Part model, mm, in its own coordinate system. Face numbers are marked on the shaded views. A direction names the side the tool comes from. Give positions to 0.01 mm unless a question says otherwise; leave off trailing zeros. Order: outer loops, then holes, each group sorted by start corner. A loop starts at its lowest first (then second) coordinate and runs counter-clockwise, first axis right, second up. Notation, with made-up numbers: M -9.5,59.25 L 16.5,59.25 A19 ccw 16.5,91.25 Z; hole C 47.5,-17.75 d5. An arc over 180 degrees is marked long. Return JSON: item names as keys, results as strings.
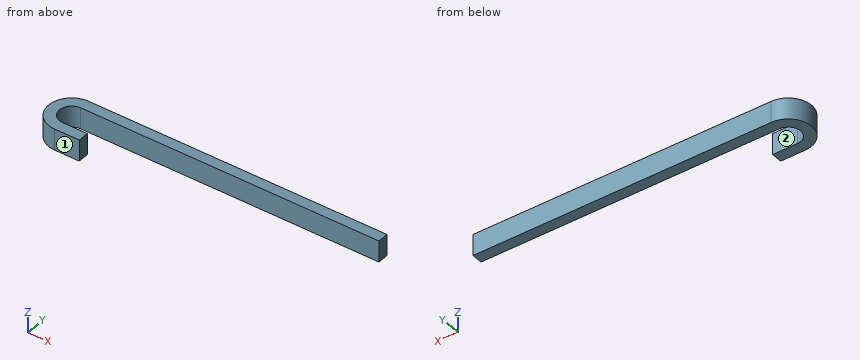
Autodesk Inventor part; units mm, degrees
ref_plane "YZ Plane" through (0, 0, 0) normal (1, 0, 0) x (0, 1, 0)
ref_plane "XZ Plane" through (0, 0, 0) normal (0, 1, 0) x (-1, 0, 0)
ref_plane "XY Plane" through (0, 0, 0) normal (0, 0, 1) x (1, 0, 0)
sketch "Sketch1" plane through (0, 0, 0) normal (0, 0, 1) x (1, 0, 0)
  circle A0 centre (0, 0) radius 42.5
  line L0 (0, -42.5) -> (45.5, -42.5)
  line L1 (45.5, -42.5) -> (45.5, -22.5)
  line L2 (45.5, -22.5) -> (0, -22.5)
  line L3 (0, -22.5) -> (0, -42.5)
  line L4 (0, 42.5) -> (550, 42.5)
  line L5 (550, 42.5) -> (550, 22.5)
  line L6 (550, 22.5) -> (0, 22.5)
  line L7 (0, 22.5) -> (0, 42.5)
  circle A1 centre (0, 0) radius 22.5
  point P0 (0, -22.5)
  point P1 (0, 22.5)
  point P2 (15.5, -22.5)
  point P3 (-42.5, 0)
  dimension "d0" = 85
  dimension "d1" = 20
  dimension "d2" = 20
  dimension "d9" = 550
  dimension "d10" = 58
  dimension "d11" = 30
extrude "Extrusion1" add sketch "Sketch1" along normal blind 39 contours L7 A1 L3 A0 | L4 L5 L6 A0 | A0 L6 L7 | L3 L2 A0 | A0 L2 L1 L0
properties part number "J15BF.1.30_Zaxis"
Q1. Band-saw the part on B-B (z = 33). Give the cut face in (x, y).
Established:
{"outline": "M 0,-42.5 L 45.5,-42.5 L 45.5,-22.5 L 0,-22.5 A22.5 cw 0,22.5 L 550,22.5 L 550,42.5 L 0,42.5 A42.5 ccw Z"}
Q2. Pin check, flat tips, straight feed: pin 1 (19.5 mm diameter, centred on x = 265.5, z = 16, fed in from -Y); pin 2 (1.5 mm diameter, centred on y = -15.5, z = 7.5, fed in from -X); pin 3 (6 mm diameter, centred on y = -36, z = 15, fed in from +X). Stop position of each tip, or through.
Established:
{"pin 1": "stops at y = 22.5", "pin 2": "stops at x = -39.86", "pin 3": "stops at x = 45.5"}
Q3. Band-saw the part on D-D (x = 162). Give the cut face in (y, z).
Established:
{"outline": "M 22.5,0 L 42.5,0 L 42.5,39 L 22.5,39 Z"}
Q4. Band-saw the part on C-C (y = 0). Give the cut face in (x, z), then the cut area to 3 significant figures.
Established:
{"outline": "M -42.5,0 L -22.5,0 L -22.5,39 L -42.5,39 Z", "area": "780 mm²"}
Q5. Probe line 1 along Y through (x, z) = (13.5, 31.5); line 2 along Y through (x, z) = (343.5, 3); line 3 along X through (y, z) = (19, 22). List the from-to ranges inside material, lowest first.
Established:
{"line 1": "y = -42.5 to -22.5, 22.5 to 42.5", "line 2": "y = 22.5 to 42.5", "line 3": "x = -38.02 to -12.05"}
Q6. Band-saw the part on A-A (x = 35.5). Give the cut face in (y, z), then the cut area to 3 significant figures.
Established:
{"outline": "M -42.5,0 L -22.5,0 L -22.5,39 L -42.5,39 Z; M 22.5,0 L 42.5,0 L 42.5,39 L 22.5,39 Z", "area": "1,560 mm²"}
Q7. 3-axis set-ups, long thin cutter, end or side, ignore diameter. For the marked faces 1 and 2: which of +Z, -Z, +X, -X, +Y, -Y reach the whole face in a straight line?
Established:
{"face 1": "+Z, -Z, +X, -X, -Y", "face 2": "+Z, -Z, +X"}
